Geometry check sheet. Reference: the model listing, model coordinates, mm. Face numbers are marked on the shaded views. Coordinates: 2 decimals unless noted, no trailing zeros. Write each loop counter-clockwise with the first axis right and the second up, starting at its lowest first coordinate (ties: lowest second). Pieces come first, ordered by that corner, then holes. Notation, with made-up numbers: (-39, 58.5) -> (9, 58.5) arc R22 cw to (9, 68.5) -> close; hole circle Ø8 at (47, -30.75). An arc over 180 degrees is marked (long way). Answer in a Markdown table with one row per item. Add a question column.
Q1. Thickness scan on line 1 (Y direction, x = 45, z = 0.75) (3 decimals); line 2 (Y direction, x = -11.25, z = 6.75); line 3 (Y direction, x = 14.5, z = 2). Record the ranges inside material, lowest first.
Q2. Release check for a two-part mould opening along X. For the marked faces 1 and 2 record: pulls with the +X half, pulls with the -X half, needs draft (parallel to the pull), parting line crosses it, or undercut.
Q3. Section check B-B, the plane x = -11.25. Record the boundary of the cut face in (y, z).
Q4. Section check D-D, the plane x = -40.5. Record the boundary of the cut face in (y, z), and give its area (3 significant figures).
Q5. Gauge pin test, flat ends, axial feed: P1, Ø4.5, axis at x = -11.25, y = 26.25, coming from the -Z side; P2, Ø1.6, axis at x = -35, y = -47, coming from the +Z side; P3, Ø5, axis at x = 14, z = 7, coming from the +Y side; P4, Ø3, axis at y = -18, z = 7, coming from the -X side. Record the tip position at first contact, or that the pin passes through.
Q6. Section check C-C, the plane y = -32. Record the boundary of the cut face in (x, z), and give its area (3 significant figures).
Q7. Section check A-A, the plane y = 26.25. Record the boundary of the cut face in (x, z), and give its area (3 significant figures).
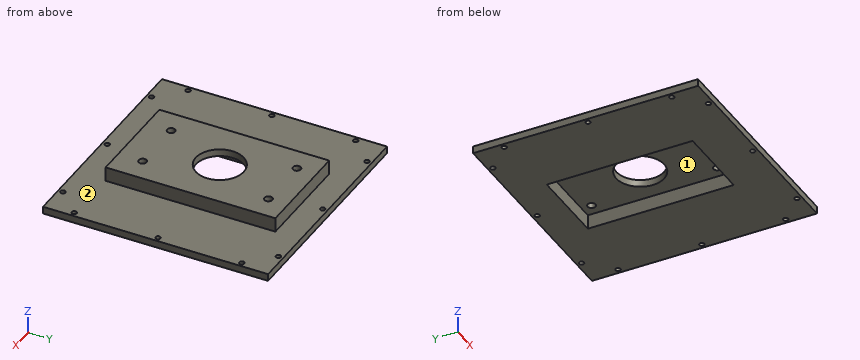
```python
from build123d import *

# Parameters (mm, degrees)
SKETCH_1_W               = 94
SKETCH_1_H               = 94
SKETCH_1_W_2             = 42.5
SKETCH_1_H_2             = 70.9
EXTRUDE_1_DEPTH          = 3
SKETCH_1_5_W             = 42.5
SKETCH_1_5_H             = 70.9
SKETCH_1_5_W_2           = 32.5
SKETCH_1_5_H_2           = 60.9
EXTRUDE_2_DEPTH          = 6
SKETCH_2_W               = 42.5
SKETCH_2_H               = 70.9
SKETCH_2_R               = 10
EXTRUDE_3_DEPTH          = 3
HOLE_WIZARD_M4_1_D       = 3.3
HOLE_WIZARD_M4_1_DEPTH   = 11.5
HOLE_WIZARD_M4_1_TIP     = 0.991420021
HOLE_WIZARD_M2_5_1_D     = 2.05
HOLE_WIZARD_M2_5_1_DEPTH = 7.25
HOLE_WIZARD_M2_5_1_TIP   = 0.615882135
HOLE_WIZARD_M2_5_2_D     = 2.05
HOLE_WIZARD_M2_5_2_DEPTH = 7.25
HOLE_WIZARD_M2_5_2_TIP   = 0.615882135


with BuildPart() as part:
    # 草图1 → 凸台-拉伸1 (new body)
    with BuildSketch(Plane.XY):
        with Locations((0, -2)):
            Rectangle(SKETCH_1_W, SKETCH_1_H)
        with Locations((0, -1)):
            Rectangle(SKETCH_1_W_2, SKETCH_1_H_2, mode=Mode.SUBTRACT)
    extrude(amount=EXTRUDE_1_DEPTH)

    # 草图1<5> → 凸台-拉伸2 (add)
    with BuildSketch(Plane.XY):
        with Locations((0, -1)):
            Rectangle(SKETCH_1_5_W, SKETCH_1_5_H)
        Rectangle(SKETCH_1_5_W_2, SKETCH_1_5_H_2, mode=Mode.SUBTRACT)
    extrude(amount=EXTRUDE_2_DEPTH)

    # 草图2 → 凸台-拉伸3 (add)
    with BuildSketch(Plane.XY.offset(6)):
        with Locations((0, -1)):
            Rectangle(SKETCH_2_W, SKETCH_2_H)
        Circle(SKETCH_2_R, mode=Mode.SUBTRACT)
    extrude(amount=EXTRUDE_3_DEPTH)

    # M4 螺纹孔1
    with Locations(Plane.XY.offset(9)):
        with Locations((11.25, 26.25), (-11.25, 26.25), (-11.25, -26.25), (11.25, -26.25)):
            Hole(HOLE_WIZARD_M4_1_D / 2, depth=HOLE_WIZARD_M4_1_DEPTH)
            with Locations((0, 0, -(HOLE_WIZARD_M4_1_DEPTH + HOLE_WIZARD_M4_1_TIP / 2))):  # 118° drill point
                Cone(0, HOLE_WIZARD_M4_1_D / 2, HOLE_WIZARD_M4_1_TIP, mode=Mode.SUBTRACT)

    # M2.5 螺纹孔1
    with Locations(Plane.XY.offset(3)):
        with Locations((-45, 33), (-45, -2), (-45, -37), (-35, 43), (0, 43), (35, 43), (45, 33)):
            Hole(HOLE_WIZARD_M2_5_1_D / 2, depth=HOLE_WIZARD_M2_5_1_DEPTH)
            with Locations((0, 0, -(HOLE_WIZARD_M2_5_1_DEPTH + HOLE_WIZARD_M2_5_1_TIP / 2))):  # 118° drill point
                Cone(0, HOLE_WIZARD_M2_5_1_D / 2, HOLE_WIZARD_M2_5_1_TIP, mode=Mode.SUBTRACT)

    # M2.5 螺纹孔2
    with Locations(Plane.XY.offset(3)):
        with Locations((45, -2), (45, -37), (35, -47), (0, -47), (-35, -47)):
            Hole(HOLE_WIZARD_M2_5_2_D / 2, depth=HOLE_WIZARD_M2_5_2_DEPTH)
            with Locations((0, 0, -(HOLE_WIZARD_M2_5_2_DEPTH + HOLE_WIZARD_M2_5_2_TIP / 2))):  # 118° drill point
                Cone(0, HOLE_WIZARD_M2_5_2_D / 2, HOLE_WIZARD_M2_5_2_TIP, mode=Mode.SUBTRACT)


solid = part.part
```
Calculated:
| question | item | result |
|---|---|---|
| 1 | line 1 | y = -49 to -38.025, -35.975 to -3.025, -0.975 to 31.975, 34.025 to 45 |
| 1 | line 2 | y = -36.45 to -27.9, -24.6 to 24.6, 27.9 to 34.45 |
| 1 | line 3 | y = -49 to -30.45, 30.45 to 45 |
| 2 | face 1 | undercut |
| 2 | face 2 | needs draft |
| 3 | outline | (-49, 0) -> (-30.45, 0) -> (-30.45, 6) -> (-27.9, 6) -> (-27.9, 9) -> (-36.45, 9) -> (-36.45, 3) -> (-49, 3) -> close; (-24.6, 6) -> (24.6, 6) -> (24.6, 9) -> (-24.6, 9) -> close; (27.9, 6) -> (30.45, 6) -> (30.45, 0) -> (45, 0) -> (45, 3) -> (34.45, 3) -> (34.45, 9) -> (27.9, 9) -> close |
| 4 | outline | (-49, 0) -> (45, 0) -> (45, 3) -> (-49, 3) -> close |
| 4 | area | 282 mm² |
| 5 | P1 | stops at z = 6 |
| 5 | P2 | passes through |
| 5 | P3 | stops at y = 34.45 |
| 5 | P4 | stops at x = -21.25 |
| 6 | outline | (-47, 0) -> (47, 0) -> (47, 3) -> (21.25, 3) -> (21.25, 9) -> (-21.25, 9) -> (-21.25, 3) -> (-47, 3) -> close |
| 6 | area | 537 mm² |
| 7 | outline | (-47, 0) -> (-16.25, 0) -> (-16.25, 6) -> (-12.9, 6) -> (-12.9, 9) -> (-21.25, 9) -> (-21.25, 3) -> (-47, 3) -> close; (-9.6, 6) -> (9.6, 6) -> (9.6, 9) -> (-9.6, 9) -> close; (12.9, 6) -> (16.25, 6) -> (16.25, 0) -> (47, 0) -> (47, 3) -> (21.25, 3) -> (21.25, 9) -> (12.9, 9) -> close |
| 7 | area | 322 mm² |
